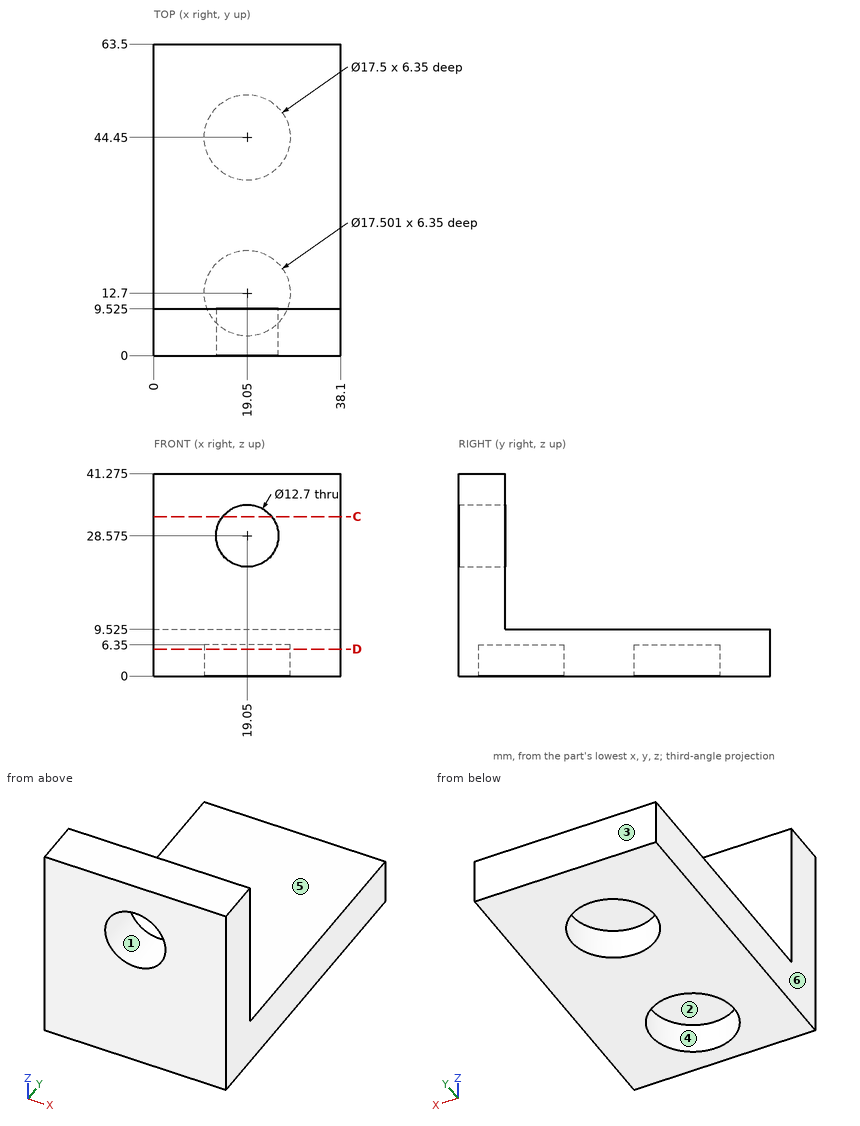
Answer from the drawing. Dimensions are ordinates in mm from the lowest x, y and z of the part. A direction names the side the tool comes from. Round coordinates to 2 decimals unless told otherwise and drop trailing zeros. Loops run counter-clockwise (first coordinate to the right, second up) from the corner with the lowest first, then second, coordinate; pieces in that order, holes last. Notation, with made-up numbers: (43.5, 63.5) - (56.5, 63.5) arc R26 cw to (56.5, 94.5) - close; hole circle Ø11 at (-23, 89). An arc over 180 degrees is marked (long way). Return JSON: item names as keys, results as strings. Group by question number.
1. The part is cut by section D-D on z = 5.5. Determine the outline of the cut face in (x, y).
2. Consider probe 1 along Y at (x, z) = (19.05, 4.5); probe 2 along Y at (x, z) = (22.5, 5); probe 3 along Y at (x, z) = (28, 23) (1 decimal). Determine where each line is inside the solid, lowest interval first.
3. Each of these flat-tipped pins is pushed along its axis until it touches: P1, Ø16.5, axis at x = 19.05, z = 28.575, coming from the +Y side (3 decimals); P2, Ø2, axis at x = 25.5, y = 44, coming from the +Z side (3 decimals); P3, Ø9, axis at x = 21, y = 13.5, coming from the -Z side. Where does it stop, or does it pass through?
4. The part is cut by section C-C on z = 32.5. Determine the outline of the cut face in (x, y) (1 decimal), then the cut area to 3 significant figures.
5. Which of the six approach directions +Z, -Z, +X, -X, +Y, -Y give full straight-line access (tool end or side, diameter ignored) to the marked faces 4, 5 and 6?
6. The mould has two halves that part along Z. Classify the marked faces 1, 2 and 3: pulls with the +Z half, pulls with the -Z half, needs draft (parallel to the pull), parting line crosses it, or undercut.
Resolved:
{
 "1": {"outline": "(0, 0) - (38.1, 0) - (38.1, 63.5) - (0, 63.5) - close; hole circle Ø17.5 at (19.05, 12.7); hole circle Ø17.5 at (19.05, 44.45)"},
 "2": {"probe 1": "y = 0 to 3.95, 21.45 to 35.7, 53.2 to 63.5", "probe 2": "y = 0 to 4.66, 20.74 to 36.41, 52.49 to 63.5", "probe 3": "y = 0 to 9.5"},
 "3": {"P1": "stops at y = 9.525", "P2": "stops at z = 9.525", "P3": "stops at z = 6.35"},
 "4": {"outline": "(0, 0) - (14.1, 0) - (14.1, 9.5) - (0, 9.5) - close; (24, 0) - (38.1, 0) - (38.1, 9.5) - (24, 9.5) - close", "area": "268 mm²"},
 "5": {"face 4": "-Z", "face 5": "+Z, +X, -X, +Y", "face 6": "+Z, -Z, -X, +Y, -Y"},
 "6": {"face 1": "undercut", "face 2": "pulls with the -Z half", "face 3": "needs draft"}
}
